from build123d import *

# Parameters (mm, degrees)
SKETCH_R        = 2.1
SKETCH_R_2      = 1.5
PAD_DEPTH       = 10
POCKET_DEPTH    = 2.5
SKETCH002_R     = 2.1
SKETCH002_R_2   = 1.5
PAD001_DEPTH    = 2
SKETCH003_R     = 3.6
SKETCH003_R_2   = 2.1
POCKET001_DEPTH = 2.5
FILLET_R        = 1
FILLET001_R     = 5
SKETCH004_R     = 1.5
PAD002_DEPTH    = 0.1


with BuildPart() as part:
    # Sketch → Pad (new body)
    with BuildSketch(Plane.XY):
        with BuildLine():
            Line((-22.5, 10), (22.5, 10))
            Line((22.5, 10), (22.5, -10))
            Line((22.5, -10), (11, -10))
            Line((11, -15), (11, -10))
            ThreePointArc((-1, -15), (5, -21), (11, -15))
            Line((-1, -15), (-1, -10))
            Line((-22.5, -10), (-1, -10))
            Line((-22.5, -10), (-22.5, 10))
        make_face()
        with Locations((-15, 0)):
            Circle(SKETCH_R, mode=Mode.SUBTRACT)
        with Locations((15, 0)):
            Circle(SKETCH_R, mode=Mode.SUBTRACT)
        with Locations((-5, 5)):
            Circle(SKETCH_R_2, mode=Mode.SUBTRACT)
        with Locations((5, -15)):
            Circle(SKETCH_R_2, mode=Mode.SUBTRACT)
    extrude(amount=PAD_DEPTH)

    # Sketch001 → Pocket (cut)
    with BuildSketch(Plane.XY.offset(10)):
        Polygon((-3.412287, 2.25), (-1.824574, 5), (-3.412287, 7.75), (-6.587713, 7.75), (-8.175426, 5), (-6.587713, 2.25), align=None)
        Polygon((6.587713, -17.75), (8.175426, -15), (6.587713, -12.25), (3.412287, -12.25), (1.824574, -15), (3.412287, -17.75), align=None)
    extrude(amount=-POCKET_DEPTH, mode=Mode.SUBTRACT)

    # Sketch002 → Pad001 (new body)
    with BuildSketch(Plane(origin=(0, 0, 0), x_dir=(1, 0, 0), z_dir=(0, 0, -1))):
        with Locations((-5, -5)):
            Circle(SKETCH002_R)
        with Locations((-5, -5)):
            Circle(SKETCH002_R_2, mode=Mode.SUBTRACT)
        with Locations((5, 15)):
            Circle(SKETCH002_R)
        with Locations((5, 15)):
            Circle(SKETCH002_R_2, mode=Mode.SUBTRACT)
    extrude(amount=PAD001_DEPTH)

    # Sketch003 → Pocket001 (cut)
    with BuildSketch(Plane(origin=(0, 0, 0), x_dir=(1, 0, 0), z_dir=(0, 0, -1))):
        with Locations((15, 0)):
            Circle(SKETCH003_R)
        with Locations((15, 0)):
            Circle(SKETCH003_R_2, mode=Mode.SUBTRACT)
        with Locations((-15, 0)):
            Circle(SKETCH003_R)
        with Locations((-15, 0)):
            Circle(SKETCH003_R_2, mode=Mode.SUBTRACT)
    extrude(amount=-POCKET001_DEPTH, mode=Mode.SUBTRACT)

    # Fillet
    fillet_edges = [part.edges().sort_by_distance(p)[0] for p in [
        (2.9, -15, 0),
        (-7.1, 5, 0),
    ]]
    fillet(fillet_edges, radius=FILLET_R)

    # Fillet001
    fillet001_edges = [part.edges().sort_by_distance(p)[0] for p in [
        (22.5, 10, 5),
        (22.5, -10, 5),
        (-22.5, 10, 5),
        (-22.5, -10, 5),
    ]]
    fillet(fillet001_edges, radius=FILLET001_R)

    # Sketch004 → Pad002 (new body)
    with BuildSketch(Plane.XY.offset(7.5)):
        with Locations((-5, 5)):
            Circle(SKETCH004_R)
        with Locations((5, -15)):
            Circle(SKETCH004_R)
    extrude(amount=-PAD002_DEPTH)


solid = part.part
Work out the finished part from the listing and answer in its coordinate system (mm). A direction names the side the tool comes from. Round coordinates to 2 decimals unless told otherwise and drop trailing zeros. Loops run counter-clockwise (first coordinate to the right, second up) from the corner with the lowest first, then second, coordinate; pieces in that order, holes last. Notation, with made-up numbers: (41, -9.75) - (58, -9.75) arc R15 cw to (58, 15.25) - close; hole circle Ø3 at (36.25, 54). An arc over 180 degrees is marked (long way). One line per item, written item: value.
Q1. The mould has two halves that part along Y. Classify faces 1 (the flat face through (17, 2, 2.5)), 2 (the flat face through (-22.5, 0, 5)), 3 (the cylindrical face through (5, -21, 5)): +Y half, -Y half, draft (parallel to the pull), parting line (faces both ways), or undercut.
Check values:
face 1: undercut
face 2: draft
face 3: -Y half
Q2. Find section A-A on x = 15. Give the vertices of the cut face in (y, z), and give its area (4 significant figures).
Check values:
outline: (-10, 0) - (-3.6, 0) - (-3.6, 2.5) - (-2.1, 2.5) - (-2.1, 10) - (-10, 10) - close; (2.1, 2.5) - (3.6, 2.5) - (3.6, 0) - (10, 0) - (10, 10) - (2.1, 10) - close
area: 150.5 mm2
Q3. Find section B-B on z = 3.75. Give the vertices of the cut face in (x, y), and give its area (3 significant figures).
Check values:
outline: (-22.5, -5) arc R5 ccw to (-17.5, -10) - (-1, -10) - (-1, -15) arc R6 ccw to (11, -15) - (11, -10) - (17.5, -10) arc R5 ccw to (22.5, -5) - (22.5, 5) arc R5 ccw to (17.5, 10) - (-17.5, 10) arc R5 ccw to (-22.5, 5) - close; hole circle Ø4.2 at (-15, 0); hole circle Ø3 at (-5, 5); hole circle Ø3 at (5, -15); hole circle Ø4.2 at (15, 0)
area: 953 mm2
Q4. Straight lines are drawn through the part: probe 1 along X at (y, z) = (0, 4); probe 2 along Y at (x, z) = (-5, -1); probe 3 along X at (y, z) = (-15, 6). For each, find the intervals that lie inside material, in ascending order.
Check values:
probe 1: -22.5 to -17.1, -12.9 to 12.9, 17.1 to 22.5
probe 2: 2.9 to 3.5, 6.5 to 7.1
probe 3: -1 to 3.5, 6.5 to 11
Q5. For faces 4 (the cylindrical face through (-5.46, 7.05, -1.49)), 5 (the flat face through (-1, -13, 5)), 6 (the flat face through (0, 10, 5)), 7 (the flat face through (-3.6, 5.9, -2)), 8 (the flat face through (-7.39, 3.64, 8.77)), determine the directions among +Z, -Z, +X, -X, +Y, -Y from which every point of the face is accessible in a straight line to the end or side of a thin tool.
Check values:
face 4: -Z
face 5: +Z, -Z, -X, -Y
face 6: +Z, -Z, +X, -X, +Y
face 7: -Z, +X, -X, +Y, -Y
face 8: +Z
Q6. Each of these flat-tipped pins is pushed along its axis until it touches: pin 1 Ø2.5 at (x, y) = (5, -15) entering from -Z; pin 2 Ø4 at (y, z) = (-13.5, 4.5) entering from -X; pin 3 Ø6 at (y, z) = (-12.5, 0.5) entering from -X. Where does it stop, or does it pass through?
Check values:
pin 1: z = 7.4
pin 2: x = -1
pin 3: x = -19.68
Q7. Find section C-C on x = 5. Give the vertices of the cut face in (y, z), and give its area (3 significant figures).
Check values:
outline: (-21, 0) - (-18.1, 0) arc R1 cw to (-17.1, -1) - (-17.1, -2) - (-16.5, -2) - (-16.5, 7.4) - (-13.5, 7.4) - (-13.5, -2) - (-12.9, -2) - (-12.9, -1) arc R1 cw to (-11.9, 0) - (10, 0) - (10, 10) - (-12.25, 10) - (-12.25, 7.5) - (-17.75, 7.5) - (-17.75, 10) - (-21, 10) - close
area: 277 mm2
Q8. Find section D-D on y = -4.5. Give the vertices of the cut face in (x, z), and give its area (3 significant figures).
Check values:
outline: (-22.5, 0) - (22.5, 0) - (22.5, 10) - (-22.5, 10) - close
area: 450 mm2
